Check sheet for the modelled part. Datum: model origin and axes. Units: mm. Give positions to 0.01 mm unless a question says otherwise; leave off trailing zeros. Order: outer loops, then holes, each group sorted by start corner. A loop starts at its lowest first (then second) coordinate and runs counter-clockwise, first axis right, second up.
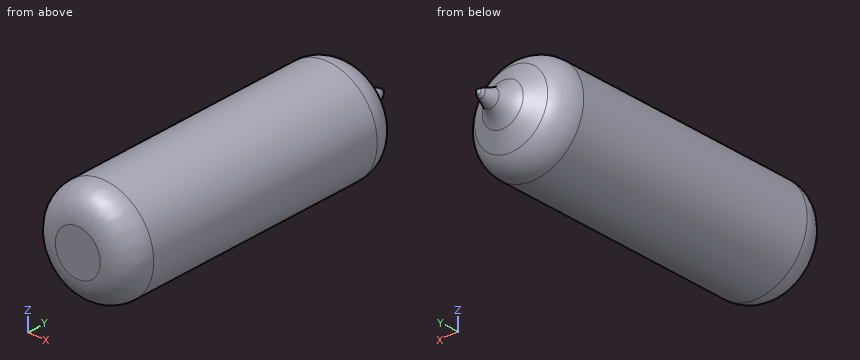
```python
from build123d import *


with BuildPart() as part:
    # Esquisse1 → Révolution1 (revolve)
    with BuildSketch(Plane.XY):
        with BuildLine():
            Line((-3.902413526, 31.860615398), (-2.193843177, 32.849176927))
            ThreePointArc((-2.193843177, 32.849176927), (-1.444814591, 33.46318111), (-0.930447552, 34.283834209))
            Line((-0.930447552, 34.283834209), (-0.459450443, 35.40488518))
            ThreePointArc((-0.459450443, 35.40488518), (-0.382581088, 35.552204227), (-0.282377912, 35.684760339))
            Line((-0.282377912, 35.684760339), (0, 36))
            Line((0, 36), (0, 0))
            Line((0, 0), (-2.4, 0))
            ThreePointArc((-2.4, 0), (-4.521320344, 0.878679656), (-5.4, 3))
            Line((-5.4, 3), (-5.4, 29.263934132))
            ThreePointArc((-5.4, 29.263934132), (-4.998772843, 30.762726883), (-3.902413526, 31.860615398))
        make_face()
    revolve(axis=Axis((0, 36, 0), (0, -1, 0)))


solid = part.part
```
Q1. Material ranges on line 1 (Y direction, x = 1.75, z = 4.75); line 2 (X direction, y = 7, z = -3.5); line 3 (X direction, y = 20.5, z = 2.5), recorded low to high.
Q2. Sectioned sample at B-B, the plane y = 33.5. Record the cut outline in (x, z), plus the area to 3 significant figures.
Q3. Sectioned sample at A-A, the plane y = 18.5. Record the cut outline in (x, z).
Q4. Go/stop test with flat-tipped pins: P1, Ø1.5, axis at x = -1.5, z = -0.5, coming from the +Y side; P2, Ø2, axis at x = -3.5, z = -3.5, coming from the +Y side; P3, Ø2, axis at x = -1, z = 0.5, coming from the +Y side. Record where each tip stops, or that it passes through.
Filled in:
1. line 1: y = 1.62 to 30.65
1. line 2: x = -4.11 to 4.11
1. line 3: x = -4.79 to 4.79
2. outline: circle Ø2.83 at (0, 0)
2. area: 6.27 mm2
3. outline: circle Ø10.8 at (0, 0)
4. P1: stops at y = 34.52
4. P2: stops at y = 31.83
4. P3: stops at y = 35.87
